Model file for the job. Use its own axes, mm. A direction names the side the tool comes from. Coordinates: 2 decimals unless noted, no trailing zeros. Order: outer loops, then holes, each group sorted by start corner. A loop starts at its lowest first (then second) coordinate and runs counter-clockwise, first axis right, second up. Notation, with made-up numbers: (19.25, -25.5) -> (37.25, -25.5) arc R20 ccw to (37.25, -21.5) -> close; hole circle Ø4 at (75, 49). An arc over 180 degrees is marked (long way). Return JSON: item names as keys, results as strings. Group by question number.
1) Cut at B-B (y = 88.9). Write the cut outline in (x, z).
2) Cut at D-D (x = 26). Write the cut outline in (y, z).
3) Flat gauge pins, fed straight in: pin 1 (8.5 mm diameter, centred on x = 0, y = 88.9, fed in from +Z); pin 2 (1.5 mm diameter, centred on x = -27.5, z = -4, fed in from -Y); pin 3 (2.5 mm diameter, centred on x = -1.5, z = 2, fed in from -Y). Where does each tip first touch, or does it go through?
4) Which spindle directions (+Z, -Z, +X, -X, +Y, -Y) get a long thin tool onto all of the face, cutting with end or side? Do faces 1 (the flat face through (38.1, 1, 0)), 2 (the flat face through (0, 6.604, 0)). Say none if no direction does.
5) Cut at A-A (x = 0). Write the cut outline in (y, z).
6) Cut at C-C (z = -4.25). Write the cut outline in (x, y).
7) Pull direction X, two halves, no side cores. Call faces 3 (the flat face through (-9, 1, 6.35)), 4 (the flat face through (-5.69, -3.35, -0.09)), 5 (the cylindrical face through (0.5, -101.6, -0.1)), 6 (the flat face through (-38.1, 1, 0)): +X half, -X half, draft (parallel to the pull), parting line (faces both ways), or undercut.
8) Probe line 1 (Y direction, x = -32, z = -4.75); line 2 (Y direction, x = -18.5, z = 1.5). List the from-to ranges inside material, lowest first.
Autodesk Inventor part; units mm, degrees
ref_plane "YZ Plane" through (0, 0, 0) normal (1, 0, 0) x (0, 1, 0)
ref_plane "XZ Plane" through (0, 0, 0) normal (0, 1, 0) x (-1, 0, 0)
ref_plane "XY Plane" through (0, 0, 0) normal (0, 0, 1) x (1, 0, 0)
sketch "Sketch1" plane through (0, 0, 0) normal (0, 0, 1) x (1, 0, 0)
  circle A0 centre (0, 0) radius 101.6
  line L0 (7.6256, 0) -> (3.8128, -6.604)
  line L1 (3.8128, -6.604) -> (-3.8128, -6.604)
  line L2 (-3.8128, -6.604) -> (-7.6256, 0)
  line L3 (-7.6256, 0) -> (-3.8128, 6.604)
  line L4 (-3.8128, 6.604) -> (3.8128, 6.604)
  line L5 (3.8128, 6.604) -> (7.6256, 0)
  circle A1 centre (0, 88.9) radius 5.2705
  dimension "d0" = 203.2
  dimension "d1" = 13.208
  dimension "d2" = 10.541
  dimension "d5" = 88.9
extrude "Extrusion1" add sketch "Sketch1" along normal mid plane 12.7
sketch "Sketch4" plane through (0, 0, 6.35) normal (0, 0, 1) x (1, 0, 0)
  circle A0 centre (0, 0) radius 101.6
  line L0 (-38.1, 94.1857) -> (-38.1, -94.1857)
  line L1 (38.1, 94.1857) -> (38.1, -94.1857)
  arc A1 (-38.1, 94.1857) -> (-38.1, -94.1857) centre (0, 0) ccw
  arc A2 (38.1, -94.1857) -> (38.1, 94.1857) centre (0, 0) ccw
  dimension "d18" = 38.1
  dimension "d19" = 38.1
extrude "Extrusion4" cut sketch "Sketch4" against normal through all contours A0 L1 | L0 A0
sketch "Sketch2" plane through (0, 0, 6.35) normal (0, 0, 1) x (1, 0, 0)
  circle A0 centre (-63.5, 0) radius 25.4
  circle A1 centre (-31.75, -54.9926) radius 25.4
  circle A2 centre (31.75, -54.9926) radius 25.4
  circle A3 centre (63.5, 0) radius 25.4
  circle A4 centre (31.75, 54.9926) radius 25.4
  circle A5 centre (-31.75, 54.9926) radius 25.4
  point P0 (0, 0)
  dimension "d6" = 50.8
  dimension "d7" = 63.5
  dimension "d10" = 360
properties part number "driveForPiston-7-inV03" material "PET Plastic"
Answers below:
{
 "1": {"outline": "(-38.1, -6.35) -> (-5.27, -6.35) -> (-5.27, 6.35) -> (-38.1, 6.35) -> close; (5.27, -6.35) -> (38.1, -6.35) -> (38.1, 6.35) -> (5.27, 6.35) -> close"},
 "2": {"outline": "(-98.22, -6.35) -> (98.22, -6.35) -> (98.22, 6.35) -> (-98.22, 6.35) -> close"},
 "3": {"pin 1": "passes through", "pin 2": "stops at y = -98.02", "pin 3": "stops at y = -101.6"},
 "4": {"face 1": "+Z, -Z, +X, +Y, -Y", "face 2": "+Z, -Z"},
 "5": {"outline": "(-101.6, -6.35) -> (-6.6, -6.35) -> (-6.6, 6.35) -> (-101.6, 6.35) -> close; (6.6, -6.35) -> (83.63, -6.35) -> (83.63, 6.35) -> (6.6, 6.35) -> close; (94.17, -6.35) -> (101.6, -6.35) -> (101.6, 6.35) -> (94.17, 6.35) -> close"},
 "6": {"outline": "(-38.1, -94.19) arc R101.6 ccw to (38.1, -94.19) -> (38.1, 94.19) arc R101.6 ccw to (-38.1, 94.19) -> close; hole (-7.63, 0) -> (-3.81, -6.6) -> (3.81, -6.6) -> (7.63, 0) -> (3.81, 6.6) -> (-3.81, 6.6) -> close; hole circle Ø10.54 at (0, 88.9)"},
 "7": {"face 3": "draft", "face 4": "undercut", "face 5": "parting line", "face 6": "-X half"},
 "8": {"line 1": "y = -96.43 to 96.43", "line 2": "y = -99.9 to 99.9"}
}
